Part print with two shaded views. Sizes in mm from the minimum x, y, z corner. A direction names the side the tool comes from. Round coordinates to 2 decimals unless told otherwise and drop trailing zeros. Write each loop counter-clockwise with the first axis right and the second up, starting at its lowest first coordinate (ties: lowest second). Pieces come first, ordered by that corner, then holes. Notation, with made-up numbers: (25.25, 40.5) -> (51.25, 40.5) arc R25 cw to (51.25, 57.5) -> close; hole circle Ø10 at (-13.5, 41.5). An arc over 180 degrees is marked (long way). Answer in a Markdown table with one row per item.
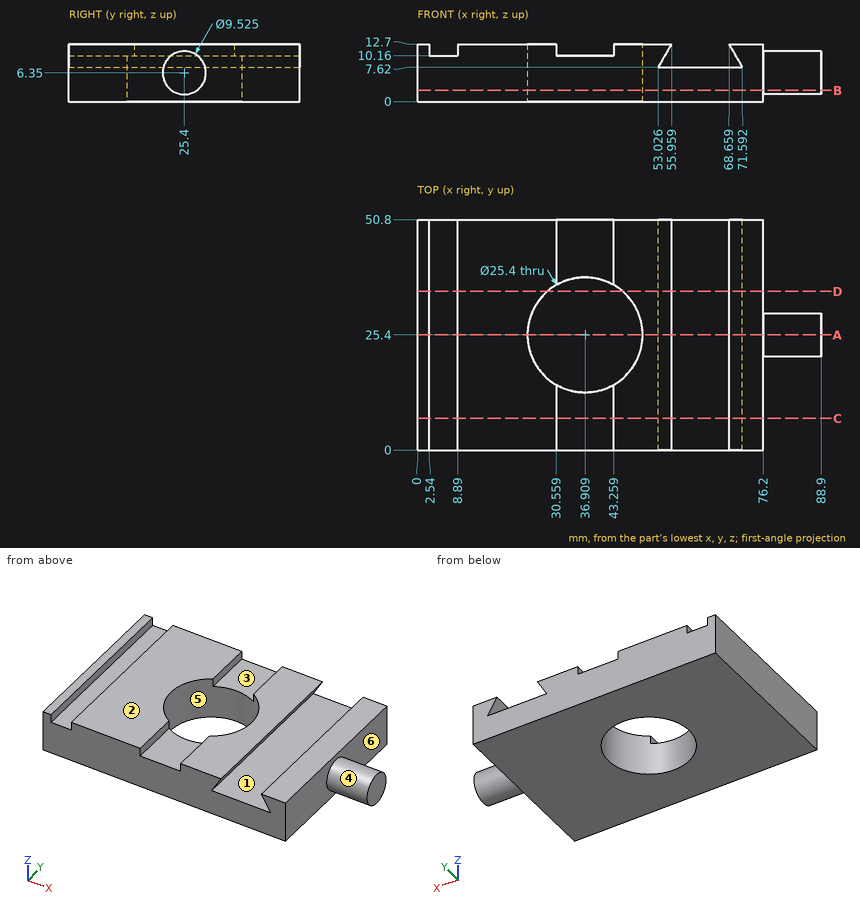
Q1. Saw through at A-A on y = 25.4. Write the cut outline in (x, z).
A:
| item | result |
|---|---|
| outline | (0, 0) -> (24.21, 0) -> (24.21, 12.7) -> (8.89, 12.7) -> (8.89, 10.16) -> (2.54, 10.16) -> (2.54, 12.7) -> (0, 12.7) -> close; (49.61, 0) -> (76.2, 0) -> (76.2, 1.59) -> (88.9, 1.59) -> (88.9, 11.11) -> (76.2, 11.11) -> (76.2, 12.7) -> (68.66, 12.7) -> (71.59, 7.62) -> (53.03, 7.62) -> (55.96, 12.7) -> (49.61, 12.7) -> close |
Q2. Saw through at D-D on y = 35. Write the cut outline in (x, z) (1 decimal), plus the area to 3 significant figures.
A:
| item | result |
|---|---|
| outline | (0, 0) -> (28.6, 0) -> (28.6, 12.7) -> (8.9, 12.7) -> (8.9, 10.2) -> (2.5, 10.2) -> (2.5, 12.7) -> (0, 12.7) -> close; (45.2, 0) -> (76.2, 0) -> (76.2, 12.7) -> (68.7, 12.7) -> (71.6, 7.6) -> (53, 7.6) -> (56, 12.7) -> (45.2, 12.7) -> close |
| area | 661 mm² |
Q3. Drop flat-ended pins along their axis: P1, Ø3, axis at y = 33.5, z = 8.5, coming from the +X side; P2, Ø1.9, axis at x = 6, y = 28, coming from the +Z side. Give the stop position or say it passes through.
A:
| item | result |
|---|---|
| P1 | x = 76.2 |
| P2 | z = 10.16 |
Q4. Wall check: line 1 (X direction, y = 25.4, z = 3); line 2 (X direction, y = 14, z = 8.75) (1 decimal); line 3 (X direction, y = 25.4, z = 9) (1 decimal). Give the ranges that are in metal, low to high. Write a range as [from, to].
A:
| item | result |
|---|---|
| line 1 | [0, 24.21], [49.61, 88.9] |
| line 2 | [0, 31.3], [42.5, 53.7], [70.9, 76.2] |
| line 3 | [0, 24.2], [49.6, 53.8], [70.8, 88.9] |
Q5. Saw through at B-B on z = 2.5. Write the cut outline in (x, y).
A:
| item | result |
|---|---|
| outline | (0, 0) -> (76.2, 0) -> (76.2, 22.6) -> (88.9, 22.6) -> (88.9, 28.2) -> (76.2, 28.2) -> (76.2, 50.8) -> (0, 50.8) -> close; hole circle Ø25.4 at (36.91, 25.4) |
Q6. Two-plate mould, pull along X, no slides. Class the marked faces 4, 5 and 6: released by +X, released by -X, zero draft, split by the parting line, or undercut.
A:
| item | result |
|---|---|
| face 4 | zero draft |
| face 5 | undercut |
| face 6 | released by +X |
Q7. Which spindle directions (+Z, -Z, +X, -X, +Y, -Y) get a long thin tool onto all of the face, cutting with end or side? Do the marked faces 1, 2 and 3. Say none if no direction does.
A:
| item | result |
|---|---|
| face 1 | +Y, -Y |
| face 2 | +Z, +X, -X, +Y, -Y |
| face 3 | +Z, +Y, -Y |
Q8. Saw through at C-C on y = 7. Write the cut outline in (x, z), plus the area to 3 significant figures.
A:
| item | result |
|---|---|
| outline | (0, 0) -> (76.2, 0) -> (76.2, 12.7) -> (68.66, 12.7) -> (71.59, 7.62) -> (53.03, 7.62) -> (55.96, 12.7) -> (43.26, 12.7) -> (43.26, 10.16) -> (30.56, 10.16) -> (30.56, 12.7) -> (8.89, 12.7) -> (8.89, 10.16) -> (2.54, 10.16) -> (2.54, 12.7) -> (0, 12.7) -> close |
| area | 840 mm² |
